CAD build for the part. Positions are in the model's coordinates, mm. A direction names the side the tool comes from. Give positions to 0.01 mm unless a question says otherwise; leave off trailing zeros. Loops run counter-clockwise (first coordinate to the right, second up) from the corner with the lowest first, then second, coordinate; pieces in that order, holes last. Notation, with made-up numbers: M 16,37.5 L 33,37.5 A19 cw 33,56.5 Z; hole C -7.5,47.5 d9. An arc over 180 degrees is marked long. Answer as CSV lines item,"result".
```python
from build123d import *

# Parameters (mm, degrees)
SKETCH137_R     = 4.6
PAD045_DEPTH    = 1.5
SKETCH138_R     = 3.9
PAD046_DEPTH    = 4
SKETCH139_R     = 1.55
POCKET092_DEPTH = 13
CHAMFER003_SIZE = 0.2


with BuildPart() as part:
    # Sketch137 → Pad045 (new body)
    with BuildSketch(Plane.XY):
        Circle(SKETCH137_R)
    extrude(amount=PAD045_DEPTH)

    # Sketch138 (on Face2 of Pad045) → Pad046 (join)
    with BuildSketch(Plane(origin=(0, 0, 0), x_dir=(1, 0, 0), z_dir=(0, 0, -1))):
        Circle(SKETCH138_R)
    extrude(amount=-PAD046_DEPTH)

    # Sketch139 (on Face4 of Pad046) → Pocket092 (cut)
    with BuildSketch(Plane.XY.offset(4)):
        Circle(SKETCH139_R)
    extrude(amount=-POCKET092_DEPTH, mode=Mode.SUBTRACT)

    # Chamfer003
    chamfer003_edges = [part.edges().sort_by_distance(p)[0] for p in [
        (-3.9, 0, 4),
        (-4.6, 0, 1.5),
    ]]
    chamfer(chamfer003_edges, length=CHAMFER003_SIZE)


solid = part.part
```
Q1. Which spindle directions (+Z, -Z, +X, -X, +Y, -Y) get a long thin tool onto all of the face, cutting with end or side? Do faces 4 (the flat face through (-3, -3, 1.5)), 5 (the cylindrical face through (-3.65, -2.8, 0.64)). Say none if no direction does.
Solution:
face 4,"+Z"
face 5,"+Z, -Z"
Q2. Mould opens along Y. For faces 1 (the cylindrical face through (-2.87, -2.64, 2.63)), 2 (the cylindrical face through (0.715, -1.375, 2.028)), 3 (the flat face through (0, 2, 0)) say: released by +Y, released by -Y, zero draft, split by the parting line, or undercut.
Solution:
face 1,"split by the parting line"
face 2,"undercut"
face 3,"zero draft"
Q3. Pin check, flat tips, straight feed: P1, Ø1, axis at x = -2, z = 3, coming from the +Y side; P2, Ø2, axis at x = -2.5, z = 1, coming from the -Y side. Stop position of each tip, or through.
Solution:
P1,"stops at y = 3.6"
P2,"stops at y = -4.35"
Q4. Cut at A-A (x = 0). Write the cut outline in (y, z).
Solution:
outline,"M -4.6,0 L -1.55,0 L -1.55,4 L -3.7,4 L -3.9,3.8 L -3.9,1.5 L -4.4,1.5 L -4.6,1.3 Z; M 1.55,0 L 4.6,0 L 4.6,1.3 L 4.4,1.5 L 3.9,1.5 L 3.9,3.8 L 3.7,4 L 1.55,4 Z"
Q5. Cut at D-D (z = 2.85). Write the cut outline in (x, y), and give its area (3 significant figures).
Solution:
outline,"C 0,0 d7.8; hole C 0,0 d3.1"
area,"40.2 mm²"
Q6. Cut at C-C (z = 0.75). Write the cut outline in (x, y), and give its area (3 significant figures).
Solution:
outline,"C 0,0 d9.2; hole C 0,0 d3.1"
area,"58.9 mm²"
Q7. Wall check: line 1 (Y direction, x = 0, z = 3.15); line 2 (Z direction, x = 0.25, y = 4); line 3 (Y direction, x = 0, z = 1.35). Give the ranges that are in metal, low to high. Write a range as [from, to].
Solution:
line 1,"y = [-3.9, -1.55], [1.55, 3.9]"
line 2,"z = [0, 1.5]"
line 3,"y = [-4.55, -1.55], [1.55, 4.55]"
